Autodesk Inventor part; units mm, degrees
ref_plane "YZ Plane" through (0, 0, 0) normal (1, 0, 0) x (0, 1, 0)
ref_plane "XZ Plane" through (0, 0, 0) normal (0, 1, 0) x (-1, 0, 0)
ref_plane "XY Plane" through (0, 0, 0) normal (0, 0, 1) x (1, 0, 0)
sketch "Sketch1" plane through (0, 0, 0) normal (0, 0, 1) x (1, 0, 0)
  line L0 (-3.175, 3.175) -> (3.175, 3.175)
  line L1 (3.175, 3.175) -> (3.175, -3.175)
  line L2 (3.175, -3.175) -> (-3.175, -3.175)
  line L3 (-3.175, -3.175) -> (-3.175, 3.175)
  point P0 (0, 0)
  dimension "d0" = 6.35
  dimension "d1" = 3.175
  dimension "d2" = 3.175
extrude "Extrusion1" add sketch "Sketch1" along normal blind 0.4064
sketch "Sketch2" plane through (-3.175, 3.175, 0) normal (0, 1, 0) x (1, 0, 0)
  line L0 (0, -0.4064) -> (6.35, -0.4064)
  line L1 (6.35, 0) -> (6.35, -0.4064)
  line L2 (0, 0) -> (6.35, 0)
  line L3 (0, 0) -> (0, -0.4064)
  line L4 (0, -0.4064) -> (6.35, -0.4064)
  line L5 (6.35, -0.4064) -> (6.35, 1.1811)
  line L6 (3.9688, 9.3726) -> (2.3812, 9.3726)
  line L7 (0, 1.1811) -> (0, -0.4064)
  line L8 (2.3812, 9.3726) -> (0, 1.1811)
  line L9 (3.9688, 9.3726) -> (6.35, 1.1811)
  point P0 (3.175, 0)
  dimension "d7" = 9.779
  dimension "d8" = 1.5875
  dimension "d9" = 1.5875
extrude "Extrusion2" add sketch "Sketch2" against normal blind 0.4064 contours L7 L8 L6 L9 L5 L2
fillet "Fillet1" radius 0.3175 1 edges at (0, 3.175, 0.4064)
fillet "Fillet2" radius 0.3175 2 edges at (-0.7938, 2.9718, -9.3726) (0.7938, 2.9718, -9.3726)
fillet "Fillet3" radius 0.3175 4 edges at (3.175, -3.175, 0.2032) (-3.175, -3.175, 0.2032) (3.175, 2.9718, -1.1811) (-3.175, 2.9718, -1.1811)
hole "Hole1" at (0, 3.175, -7.0358) direction (0, -1, 0) diameter 1.524 depth 25.4 tip angle 118
properties part number "Control_Horn"
Work out the finished part from the listing and answer in its coordinate system (mm). A direction names the side the tool comes from. Coordinates: 2 decimals unless noted, no trailing zeros. Write each loop counter-clockwise with the first axis right and the second up, starting at its lowest first coordinate (ties: lowest second). Pieces come first, ordered by that corner, then holes.
Q1. A cutting plane is placed at C-C, the plane x = -1.5. Give the vertices of the cut face in (y, z) (1 decimal).
Q2. Find the intervals of material crossed by line 1 (Z direction, x = 0, y = 2.9); line 2 (Z direction, x = -0.75, y = -0.5); line 3 (Y direction, x = -2, z = -4.75) (3 decimals), in increasing order.
Q3. Each of these flat-tipped pins is pushed along its axis until it touches: pin 1 Ø3 at (x, z) = (0, -8) entering from -Y; pin 2 Ø1 at (x, y) = (-1, 0) entering from -Z. Where does it stop, or does it pass through?
Q4. Determine the mould class of faces 3 (the face through (-1.995, 2.975, -5.24)), 4 (the face through (-0.2, 3, -6.3)), 5 (the face through (0, 3.175, -4)) for opening direction Z: released by +Z, released by -Z, zero draft, split by the parting line, or undercut.
Q5. A cutting plane is placed at B-B, the plane y = -1.75. Give the vertices of the cut face in (x, z) (3 decimals).
Q6. A cutting plane is placed at D-D, the plane z = -0.25. Give the vertices of the cut face in (x, y) (3 decimals).
Q7. A cutting plane is placed at A-A, the plane x = 0. Give the vertices of the cut face in (y, z) (1 decimal).
Q8. Which of the six approach directions +Z, -Z, +X, -X, +Y, -Y give full straight-line access (tool end or side, diameter ignored) to faces 1 (the face through (0, 2.769, -4)), 2 (the face through (1.995, 2.975, -5.24))?
Findings below:
1. outline: (-3.2, 0) - (2.8, 0) - (2.8, -6.9) - (3.2, -6.9) - (3.2, 0.1) arc R0.3 ccw to (2.9, 0.4) - (-3.2, 0.4) - close
2. line 1: z = -9.37 to -7.8, -6.27 to 0.4
2. line 2: z = 0 to 0.41
2. line 3: y = 2.769 to 3.175
3. pin 1: stops at y = 2.77
3. pin 2: stops at z = 0
4. face 3: released by -Z
4. face 4: undercut
4. face 5: zero draft
5. outline: (-3.175, 0) - (3.175, 0) - (3.175, 0.406) - (-3.175, 0.406) - close
6. outline: (-3.175, 2.769) - (3.175, 2.769) - (3.175, 3.175) - (-3.175, 3.175) - close
7. outline: (-3.2, 0) - (2.8, 0) - (2.8, -6.3) - (3.2, -6.3) - (3.2, 0.1) arc R0.3 ccw to (2.9, 0.4) - (-3.2, 0.4) - close; (2.8, -9.4) - (3.2, -9.4) - (3.2, -7.8) - (2.8, -7.8) - close
8. face 1: -Z, +X, -X, -Y
8. face 2: -Z, +X, +Y, -Y
